```python
from build123d import *

# Parameters (mm, degrees)
SKETCH1_W               = 70
SKETCH1_H               = 70
BOSS_EXTRUDE1_DEPTH     = 10
SKETCH2_R               = 12
SKETCH2_R_2             = 2
SKETCH2_R_3             = 11.5
CUT_EXTRUDE1_DEPTH      = 10
SKETCH3_W               = 10
SKETCH3_H               = 70
BOSS_EXTRUDE2_DEPTH     = 15
SKETCH4_W               = 10
SKETCH4_H               = 70
BOSS_EXTRUDE3_DEPTH     = 15
SKETCH5_R               = 11.5
SKETCH5_R_2             = 4
BOSS_EXTRUDE4_DEPTH     = 2
SKETCH6_R               = 1.5
SKETCH6_R_2             = 1.648708122
CUT_EXTRUDE3_DEPTH      = 10
BOSS_EXTRUDE5_START     = -10
SKETCH7_R               = 11.986708095
SKETCH7_R_2             = 2
BOSS_EXTRUDE5_DEPTH     = 10
SKETCH8_R               = 12
CUT_EXTRUDE4_DEPTH      = 10
SKETCH9_R               = 2
CUT_EXTRUDE5_DEPTH      = 10
CUT_EXTRUDE7_DEPTH      = 5
SKETCH15_W              = 14
SKETCH15_H              = 70
CUT_EXTRUDE8_DEPTH      = 5
CUT_EXTRUDE9_DEPTH      = 19
CUT_EXTRUDE9_DEPTH_BACK = 48
SKETCH16_R              = 1.5
SKETCH17_R              = 5
CUT_EXTRUDE10_DEPTH     = 19
SKETCH18_W              = 44.558304453
SKETCH18_H              = 39
BOSS_EXTRUDE6_DEPTH     = 5


with BuildPart() as part:
    # Sketch1 → Boss-Extrude1 (new body)
    with BuildSketch(Plane.XY):
        with Locations((35, 35)):
            Rectangle(SKETCH1_W, SKETCH1_H)
    extrude(amount=BOSS_EXTRUDE1_DEPTH)

    # Sketch2 → Cut-Extrude1 (cut)
    with BuildSketch(Plane.XY.offset(10)):
        with Locations((35, 49)):
            Circle(SKETCH2_R)
        with Locations((19.5, 65)):
            Circle(SKETCH2_R_2)
        with Locations((50.5, 65)):
            Circle(SKETCH2_R_2)
        with Locations((19.5, 34)):
            Circle(SKETCH2_R_2)
        with Locations((50.5, 34)):
            Circle(SKETCH2_R_2)
        with Locations((15, 15)):
            Circle(SKETCH2_R_3)
        with Locations((55, 15)):
            Circle(SKETCH2_R_3)
    extrude(amount=-CUT_EXTRUDE1_DEPTH, mode=Mode.SUBTRACT)

    # Sketch3 → Boss-Extrude2 (add)
    with BuildSketch(Plane.ZY):
        with Locations((5, 35)):
            Rectangle(SKETCH3_W, SKETCH3_H)
    extrude(amount=BOSS_EXTRUDE2_DEPTH)

    # Sketch4 → Boss-Extrude3 (add)
    with BuildSketch(Plane(origin=(70, 0, 0), x_dir=(0, 0, -1), z_dir=(1, 0, 0))):
        with Locations((-5, 35)):
            Rectangle(SKETCH4_W, SKETCH4_H)
    extrude(amount=BOSS_EXTRUDE3_DEPTH)

    # Sketch5 → Boss-Extrude4 (add)
    # profile 1 of 2: a face of its own
    with BuildSketch(Plane.XY.offset(10)):
        with Locations((15, 15)):
            Circle(SKETCH5_R)
        with Locations((15, 15)):
            Circle(SKETCH5_R_2, mode=Mode.SUBTRACT)
    # profile 2 of 2: a face of its own
    with BuildSketch(Plane.XY.offset(10)):
        with Locations((55, 15)):
            Circle(SKETCH5_R)
        with Locations((55, 15)):
            Circle(SKETCH5_R_2, mode=Mode.SUBTRACT)
    extrude(amount=-BOSS_EXTRUDE4_DEPTH)

    # Sketch6 → Cut-Extrude3 (cut)
    with BuildSketch(Plane(origin=(0, 0, 0), x_dir=(-1, 0, 0), z_dir=(0, 0, -1))):
        with Locations((-80, 65)):
            Circle(SKETCH6_R)
        with Locations((-80, 5)):
            Circle(SKETCH6_R)
        with Locations((10, 65)):
            Circle(SKETCH6_R_2)
        with Locations((10, 5)):
            Circle(SKETCH6_R)
    extrude(amount=-CUT_EXTRUDE3_DEPTH, mode=Mode.SUBTRACT)

    # Sketch7 → Boss-Extrude5 (add)
    with BuildSketch(Plane(origin=(0, 0, 0), x_dir=(-1, 0, 0), z_dir=(0, 0, -1)).offset(BOSS_EXTRUDE5_START)):
        with Locations((-35, 49)):
            Circle(SKETCH7_R)
        with Locations((-50.5, 65)):
            Circle(SKETCH7_R_2)
        with Locations((-19.5, 65)):
            Circle(SKETCH7_R_2)
        with Locations((-19.5, 34)):
            Circle(SKETCH7_R_2)
        with Locations((-50.5, 34)):
            Circle(SKETCH7_R_2)
    extrude(amount=BOSS_EXTRUDE5_DEPTH)


with BuildPart() as boss_extrude5_piece_1:
    # of the separate pieces the step leaves, piece 1, a body of its own (boss_extrude5_pieces)
    add(part.part.solids().sort_by_distance((-15, 0, 0))[0])


with BuildPart() as boss_extrude5_piece_2:
    # of the separate pieces the step leaves, piece 2, a body of its own (boss_extrude5_pieces)
    add(part.part.solids().sort_by_distance((23.013291905, 49, 10))[0])


with BuildPart() as cut_extrude4_tool:
    # Sketch8 → Cut-Extrude4 (new body)
    with BuildSketch(Plane(origin=(0, 0, 0), x_dir=(-1, 0, 0), z_dir=(0, 0, -1))):
        with Locations((-33.928692494, 49)):
            Circle(SKETCH8_R)
    extrude(amount=-CUT_EXTRUDE4_DEPTH)


with BuildPart() as boss_extrude5_piece_1_1:
    add(boss_extrude5_piece_1.part)

    # Cut-Extrude4: cut by cut_extrude4_tool
    add(cut_extrude4_tool.part, mode=Mode.SUBTRACT)

    # Sketch9 → Cut-Extrude5 (cut)
    with BuildSketch(Plane(origin=(0, 0, 0), x_dir=(-1, 0, 0), z_dir=(0, 0, -1))):
        with Locations((-49.428692494, 64.5)):
            Circle(SKETCH9_R)
        with Locations((-49.428692494, 33.5)):
            Circle(SKETCH9_R)
        with Locations((-18.428692494, 33.5)):
            Circle(SKETCH9_R)
        with Locations((-18.428692494, 64.5)):
            Circle(SKETCH9_R)
    extrude(amount=-CUT_EXTRUDE5_DEPTH, mode=Mode.SUBTRACT)


with BuildPart() as boss_extrude5_piece_2_1:
    add(boss_extrude5_piece_2.part)

    # Cut-Extrude4: cut by cut_extrude4_tool
    add(cut_extrude4_tool.part, mode=Mode.SUBTRACT)


with BuildPart() as cut_extrude7_tool:
    # Sketch14 → Cut-Extrude7 (new body)
    with BuildSketch(Plane(origin=(0, 0, 0), x_dir=(-1, 0, 0), z_dir=(0, 0, -1))):
        with BuildLine():
            Line((-85, 0), (-85, 70))
            Line((-85, 70), (15, 70))
            Line((15, 70), (15, 0))
            Line((15, 0), (1, 0))
            Line((1, 0), (1, 15))
            ThreePointArc((1, 15), (-15, 31), (-31, 15))
            Line((-31, 15), (-31, 0))
            Line((-31, 0), (-39, 0))
            Line((-39, 0), (-39, 15))
            ThreePointArc((-39, 15), (-55, 31), (-71, 15))
            Line((-71, 15), (-71, 0))
            Line((-71, 0), (-85, 0))
        make_face()
    extrude(amount=-CUT_EXTRUDE7_DEPTH)


with BuildPart() as boss_extrude5_piece_1_2:
    add(boss_extrude5_piece_1_1.part)

    # Cut-Extrude7: cut by cut_extrude7_tool
    add(cut_extrude7_tool.part, mode=Mode.SUBTRACT)

    # Sketch15 → Cut-Extrude8 (cut)
    with BuildSketch(Plane(origin=(0, 0, 5), x_dir=(-1, 0, 0), z_dir=(0, 0, -1))):
        with Locations((-78, 35)):
            Rectangle(SKETCH15_W, SKETCH15_H)
        with Locations((8, 35)):
            Rectangle(SKETCH15_W, SKETCH15_H)
    extrude(amount=-CUT_EXTRUDE8_DEPTH, mode=Mode.SUBTRACT)

    # Sketch16 → Cut-Extrude9 (cut, two sides: drawn at the far end of the back side and taken through both)
    with BuildSketch(Plane(origin=(0, 0, 5), x_dir=(-1, 0, 0), z_dir=(0, 0, -1)).offset(-CUT_EXTRUDE9_DEPTH_BACK)):
        with Locations((-66, 65)):
            Circle(SKETCH16_R)
        with Locations((-66, 5)):
            Circle(SKETCH16_R)
        with Locations((-4, 5)):
            Circle(SKETCH16_R)
        with Locations((-4, 65)):
            Circle(SKETCH16_R)
    extrude(amount=CUT_EXTRUDE9_DEPTH + CUT_EXTRUDE9_DEPTH_BACK, mode=Mode.SUBTRACT)

    # Sketch17 → Cut-Extrude10 (cut)
    with BuildSketch(Plane(origin=(0, 0, 8), x_dir=(-1, 0, 0), z_dir=(0, 0, -1))):
        with Locations((-15, 15)):
            Circle(SKETCH17_R)
        with Locations((-55, 15)):
            Circle(SKETCH17_R)
    extrude(amount=-CUT_EXTRUDE10_DEPTH, mode=Mode.SUBTRACT)



with BuildPart() as boss_extrude5_piece_2_2:
    add(boss_extrude5_piece_2_1.part)

    # Cut-Extrude7: cut by cut_extrude7_tool
    add(cut_extrude7_tool.part, mode=Mode.SUBTRACT)


with BuildPart() as boss_extrude5_piece_1_3:
    add(boss_extrude5_piece_1_2.part)

    add(boss_extrude5_piece_2_2.part)  # Boss-Extrude6 merges Boss-Extrude5 piece 2
    # Sketch18 → Boss-Extrude6 (add)
    with BuildSketch(Plane(origin=(0, 0, 5), x_dir=(-1, 0, 0), z_dir=(0, 0, -1))):
        with Locations((-37.279152227, 50.5)):
            Rectangle(SKETCH18_W, SKETCH18_H)
    extrude(amount=-BOSS_EXTRUDE6_DEPTH)


solid = boss_extrude5_piece_1_3.part
```
CAD build for the part. Positions are in the model's coordinates, mm. A direction names the side the tool comes from. Coordinates: 2 decimals unless noted, no trailing zeros. Order: outer loops, then holes, each group sorted by start corner. A loop starts at its lowest first (then second) coordinate and runs counter-clockwise, first axis right, second up. Notation, with made-up numbers: (17, -19) - (62, -19) arc R26 cw to (62, 18) - close; hole circle Ø4 at (3, 52.5). An arc over 180 degrees is marked (long way). Answer in a Markdown table with one row per item.
1. Slice it at A-A, the plane z = 2. List the corners of the cut face in (x, y).
Answer:
| item | result |
|---|---|
| outline | (-1, 0) - (31, 0) - (31, 15) arc R16 ccw to (-1, 15) - close; (39, 0) - (71, 0) - (71, 15) arc R16 ccw to (39, 15) - close; hole circle Ø3 at (4, 5); hole circle Ø23 at (15, 15); hole circle Ø23 at (55, 15); hole circle Ø3 at (66, 5) |
2. Slice it at D-D, the plane y = 5. List the corners of the cut face in (x, z), then the cut area to 3 significant figures.
Answer:
| item | result |
|---|---|
| outline | (-1, 0) - (2.5, 0) - (2.5, 10) - (-1, 10) - close; (5.5, 0) - (9.32, 0) - (9.32, 8) - (20.68, 8) - (20.68, 0) - (31, 0) - (31, 5) - (39, 5) - (39, 0) - (49.32, 0) - (49.32, 8) - (60.68, 8) - (60.68, 0) - (64.5, 0) - (64.5, 10) - (5.5, 10) - close; (67.5, 0) - (71, 0) - (71, 10) - (67.5, 10) - close |
| area | 438 mm² |
3. Flat gauge pins, fed straight in: P1, Ø14, axis at x = 55, y = 15, coming from the -Z side; P2, Ø1, axis at x = 40.5, y = 45, coming from the -Z side; P3, Ø2, axis at x = 28, z = 3.5, coming from the +Y side. Where does each tip first touch, or does it go through?
Answer:
| item | result |
|---|---|
| P1 | z = 8 |
| P2 | z = 5 |
| P3 | y = 25.58 |
4. Slice it at C-C, the plane z = 6. List the corners of the cut face in (x, y).
Answer:
| item | result |
|---|---|
| outline | (-1, 0) - (71, 0) - (71, 70) - (-1, 70) - close; hole circle Ø3 at (4, 5); hole circle Ø3 at (4, 65); hole circle Ø23 at (15, 15); hole circle Ø23 at (55, 15); hole circle Ø3 at (66, 5); hole circle Ø3 at (66, 65) |
5. Pull direction Y, two halves, no side cores. Call faces 1 (the face through (-1, 27, 7)), 2 (the face through (15, 31, 2)), 3 (the face through (16.08, 10.12, 8.99)): +Y half, -Y half, draft (parallel to the pull), parting line (faces both ways), or undercut.
Answer:
| item | result |
|---|---|
| face 1 | draft |
| face 2 | +Y half |
| face 3 | undercut |
6. Slice it at B-B, the plane x = 55. List the corners of the cut face in (y, z), then the cut area to 3 significant figures.
Answer:
| item | result |
|---|---|
| outline | (0, 0) - (3.5, 0) - (3.5, 8) - (10, 8) - (10, 10) - (0, 10) - close; (20, 8) - (26.5, 8) - (26.5, 0) - (31, 0) - (31, 5) - (70, 5) - (70, 10) - (20, 10) - close |
| area | 301 mm² |
7. 3-axis set-ups, long thin cutter, end or side, ignore diameter. For faces 4 (the face through (39, 7, 2)), 5 (the face through (64.57, 65.45, 7.53)), 6 (the face through (34, 0, 6)), 7 (the face through (57, 10, 8)), 8 (the face through (55, 31, 2)): which of +Z, -Z, +X, -X, +Y, -Y reach the whole face in a straight line?
Answer:
| item | result |
|---|---|
| face 4 | -Z, +Y, -Y |
| face 5 | +Z, -Z |
| face 6 | +Z, -Z, +X, -X, -Y |
| face 7 | -Z |
| face 8 | -Z, +Y |
8. Drill centre lines: L1, parallel to X at y = 65, z = 8.2; L2, parallel to Y at x = 15, z = 2.5; L3, parallel to Y at x = 55, z = 9.05. Where is each one in solid material? Low to high. Write a range as from..to.
Answer:
| item | result |
|---|---|
| L1 | -1..2.5, 5.5..64.5, 67.5..71 |
| L2 | 0..3.5, 26.5..31 |
| L3 | 0..10, 20..70 |
